The model under review builds one solid part; all positions refer to its coordinate system, in mm. Face numbers are marked on the shaded views. A direction names the side the tool comes from. Round coordinates to 2 decimals unless told otherwise and drop trailing zeros. Loops run counter-clockwise (first coordinate to the right, second up) from the corner with the lowest first, then second, coordinate; pieces in that order, holes last. Notation, with made-up numbers: M -37,84 L -28,84 A7 ccw -28,92 Z; hole C 3.25,72.5 d3. An arc over 180 degrees is marked long. Answer in a Markdown table with one row per item. Add a question column.
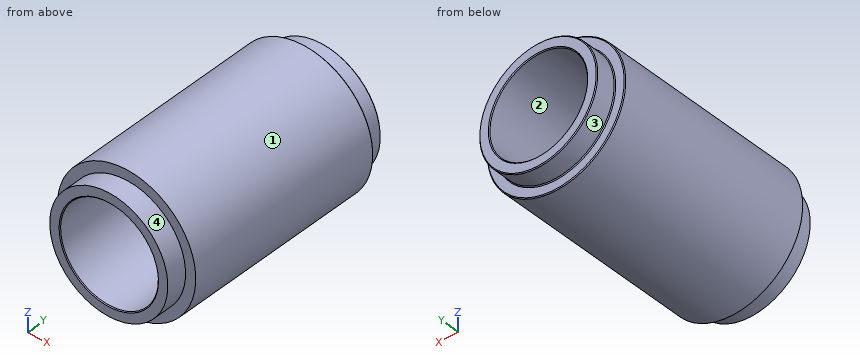
Autodesk Inventor part; units mm, degrees
ref_plane "YZ Plane" through (0, 0, 0) normal (1, 0, 0) x (0, 1, 0)
ref_plane "XZ Plane" through (0, 0, 0) normal (0, 1, 0) x (-1, 0, 0)
ref_plane "XY Plane" through (0, 0, 0) normal (0, 0, 1) x (1, 0, 0)
sketch "スケッチ1" plane through (0, 0, 0) normal (1, 0, 0) x (0, 1, 0)
  line L0 (-60, 29) -> (-50, 29)
  line L1 (-50, 29) -> (-50, 34)
  line L2 (-50, 34) -> (50, 34)
  line L3 (50, 34) -> (50, 29)
  line L4 (50, 29) -> (60, 29)
  line L5 (-60, 29) -> (-60, 24)
  line L6 (-60, 24) -> (60, 24)
  line L7 (-60, 0) -> (60, 0)
  line L8 (60, 29) -> (60, 24)
  point P0 (0, 0)
  point P1 (0, 0)
  dimension "d3" = 100
  dimension "d17" = 120
  dimension "d18" = 68
  dimension "d19" = 58
  dimension "d20" = 48
revolve "回転1" add sketch "スケッチ1" angle 360 about axis through (0, -60, 0) along (0, 1, 0)
chamfer "Chamfer1" distance 0.4 angle 45 5 edges at (0, -60, -24) (0, 60, -24) (0, 60, -29) (0, 50, -29) (0, 50, -34)
properties part number "chamber_nipple03" material "ABS Plastic"
1. To check wall thickness, follow probe 1 along X at (y, z) = (-14.5, 0); probe 2 along Y at (x, z) = (16.5, 29); probe 3 along X at (y, z) = (37, 10.5). State the ranges of each line that lie inside material, in increasing order.
2. Machinability: for the marked faces 3 and 4, which of the approach directions +Z, -Z, +X, -X, +Y, -Y give a long, thin tool a straight path to every point of the face, cutting with its end or side? Answer none if there is none.
3. Mouldability with a two-part tool opening along Z and no side actions: class the marked faces 1 and 2 as released by +Z, released by -Z, zero draft, split by the parting line, or undercut.
4. Take a section at A-A, the plane x = 0. State the section outline as (y, z) points.
5. Take a section at B-B, the plane z = 0. State the section outline as (x, y) points, and give its area (3 significant figures).
6. Take a section at C-C, the plane y = 45. State the section outline as (x, z) points.
7. For pin 1 Ø10 at (y, z) = (4, 1) entering from -X; pin 2 Ø2 at (x, y) = (22, 7) entering from +Z; pin 3 Ø6 at (y, z) = (-6, 2) entering from +X, all flat-tipped, find the tip position at first contact; note any pin that passes through.
Check sheet entries:
| question | item | result |
|---|---|---|
| 1 | probe 1 | x = -34 to -24, 24 to 34 |
| 1 | probe 2 | y = -50 to 50 |
| 1 | probe 3 | x = -32.34 to -21.58, 21.58 to 32.34 |
| 2 | face 3 | +Y |
| 2 | face 4 | -Y |
| 3 | face 1 | split by the parting line |
| 3 | face 2 | undercut |
| 4 | outline | M -60,-29 L -50,-29 L -50,-34 L 49.6,-34 L 50,-33.6 L 50,-29.4 L 50.4,-29 L 59.6,-29 L 60,-28.6 L 60,-24.4 L 59.6,-24 L -59.6,-24 L -60,-24.4 Z; M -60,24.4 L -59.6,24 L 59.6,24 L 60,24.4 L 60,28.6 L 59.6,29 L 50.4,29 L 50,29.4 L 50,33.6 L 49.6,34 L -50,34 L -50,29 L -60,29 Z |
| 5 | outline | M -34,-50 L -29,-50 L -29,-60 L -24.4,-60 L -24,-59.6 L -24,59.6 L -24.4,60 L -28.6,60 L -29,59.6 L -29,50.4 L -29.4,50 L -33.6,50 L -34,49.6 Z; M 24,-59.6 L 24.4,-60 L 29,-60 L 29,-50 L 34,-50 L 34,49.6 L 33.6,50 L 29.4,50 L 29,50.4 L 29,59.6 L 28.6,60 L 24.4,60 L 24,59.6 Z |
| 5 | area | 2,200 mm^2 |
| 6 | outline | C 0,0 d68; hole C 0,0 d48 |
| 7 | pin 1 | stops at x = -34 |
| 7 | pin 2 | stops at z = 26.74 |
| 7 | pin 3 | stops at x = 34 |
